from build123d import *

# Parameters (mm, degrees)
F0_R     = 5
F0_R_2   = 1.5
F0_R_3   = 2.5
F1_DEPTH = 5
F2_DEPTH = 45
F3_DEPTH = 4.7
F4_DEPTH = 20
F7_DEPTH = 15


with BuildPart() as f1:
    # F0 (on Front) → F1 (new body)
    with BuildSketch(Plane.XZ):
        with BuildLine():
            ThreePointArc((-17.146428, 3.5), (-16.612416, -5.502512), (-11.666667, -13.04373))
            ThreePointArc((-11.666667, -13.04373), (0, -17.5), (11.666667, -13.04373))
            ThreePointArc((11.666667, -13.04373), (16.612416, -5.502512), (17.146428, 3.5))
            ThreePointArc((17.146428, 3.5), (0, 17.5), (-17.146428, 3.5))
        make_face()
        Circle(F0_R, mode=Mode.SUBTRACT)
        with BuildLine():
            Line((-23.333333, -2.608746), (-11.666667, -13.04373))
            ThreePointArc((-11.666667, -13.04373), (-16.612416, -5.502512), (-17.146428, 3.5))
            Line((-17.146428, 3.5), (-21, 3.5))
            ThreePointArc((-21, 3.5), (-24.269603, 1.248877), (-23.333333, -2.608746))
        make_face()
        with Locations((-21, 0)):
            Circle(F0_R_2, mode=Mode.SUBTRACT)
        Circle(F0_R_3)
        with BuildLine():
            ThreePointArc((17.146428, 3.5), (16.612416, -5.502512), (11.666667, -13.04373))
            Line((11.666667, -13.04373), (23.333333, -2.608746))
            ThreePointArc((23.333333, -2.608746), (24.269603, 1.248877), (21, 3.5))
            Line((21, 3.5), (17.146428, 3.5))
        make_face()
        with Locations((21, 0)):
            Circle(F0_R_2, mode=Mode.SUBTRACT)
        Circle(F0_R)
        Circle(F0_R_3, mode=Mode.SUBTRACT)
    extrude(amount=-F1_DEPTH)

    # F0 (on Front) → F2 (join)
    with BuildSketch(Plane.XZ):
        with BuildLine():
            ThreePointArc((-17.146428, 3.5), (-16.612416, -5.502512), (-11.666667, -13.04373))
            ThreePointArc((-11.666667, -13.04373), (0, -17.5), (11.666667, -13.04373))
            ThreePointArc((11.666667, -13.04373), (16.612416, -5.502512), (17.146428, 3.5))
            ThreePointArc((17.146428, 3.5), (0, 17.5), (-17.146428, 3.5))
        make_face()
        Circle(F0_R, mode=Mode.SUBTRACT)
        Circle(F0_R)
        Circle(F0_R_3, mode=Mode.SUBTRACT)
        Circle(F0_R_3)
    extrude(amount=-F2_DEPTH)

    # F0 (on Front) → F3 (join)
    with BuildSketch(Plane.XZ):
        Circle(F0_R)
        Circle(F0_R_3, mode=Mode.SUBTRACT)
        Circle(F0_R_3)
    extrude(amount=F3_DEPTH)

    # F0 (on Front) → F4 (join)
    with BuildSketch(Plane.XZ):
        Circle(F0_R_3)
    extrude(amount=F4_DEPTH)


with BuildPart() as f1_1:
    # F5: moved
    add(f1.part.moved(Location((0, -43, 0))))

    # F6 (on Front) → F7 (join)
    with BuildSketch(Plane.XZ):
        Polygon((18.091601, 15.535572), (4.408399, 23.435572), (0.966088, 17.473313), (14.649289, 9.573313), align=None)
    extrude(amount=F7_DEPTH)


solid = f1_1.part
For this review, take the finished solid that the model builds, in its own axes (mm). A direction names the side the tool comes from. Give positions to 0.01 mm unless a question says otherwise; leave off trailing zeros. Loops run counter-clockwise (first coordinate to the right, second up) from the corner with the lowest first, then second, coordinate; pieces in that order, holes last. Notation, with made-up numbers: M 70.25,59.5 L 122.25,59.5 A21 ccw 122.25,68.5 Z; hole C 30.25,-22.75 d7. An arc over 180 degrees is marked long. Answer as a JSON object with one key per item and string values. Group by question number.
Q1. Mouldability with a two-part tool opening along X and no side actions: class faces 4 (the flat face through (9, -15, 17)), 5 (the flat face through (17.42, -40.53, -7.9)), 6 (the cylindrical face through (-22.5, -40.53, 0.07)) as +X half, -X half, draft (parallel to the pull), parting line (faces both ways), or undercut.
Q2. For probe 1 along Y at (x, z) = (6.5, -13); probe 2 along Y at (x, z) = (14, 11); probe 3 along Z at (x, y) = (21, -40), list the stretches that pass through material, from the lowest coordinate up. Write a range as [from, to].
Q3. Add section A-A on z = 0. Give the boundary of the cut face in (x, y).
Q4. Tool access review of faces 1 (the cylindrical face through (-1.08, -45.32, -4.88)), 2 (the flat face through (16.346, -7.395, 12.513)), 3 (the flat face through (19, -41, 3.5)): name each direction out of +Z, -Z, +X, -X, +Y, -Y from which nothing blocks a thin tool from reaching the whole face with its end or side.
Q5. Add section B-B on y = -14. Give the boundary of the cut face in (x, z).
Q6. Add section D-D on x = 16. Give the boundary of the cut face in (y, z), and give its area (3 significant figures).
Q7. Add section C-C on x = 0. Give the boundary of the cut face in (y, z).
Q8. Insertion check: P1, Ø1.9, axis at x = -18.5, y = -41.5, coming from the +Z side; P2, Ø4, axis at x = 21, z = 0, coming from the -Y side; P3, Ø12, axis at x = 7, y = -51.5, coming from the -Z side. Each pin has a flat end and moves straight along its axis. Give the tip position at first contact, or say it passes through.
Checked values:
{
 "1": {"face 4": "draft", "face 5": "+X half", "face 6": "undercut"},
 "2": {"probe 1": "[-43, 2]", "probe 2": "[-15, 0]", "probe 3": "[-4.7, -1.5], [1.5, 3.5]"},
 "3": {"outline": "M -24.5,-43 L -22.5,-43 L -22.5,-38 L -24.5,-38 Z; M -19.5,-43 L -5,-43 L -5,-47.7 L -2.5,-47.7 L -2.5,-63 L 2.5,-63 L 2.5,-47.7 L 5,-47.7 L 5,-43 L 19.5,-43 L 19.5,-38 L 17.5,-38 L 17.5,2 L -17.5,2 L -17.5,-38 L -19.5,-38 Z; M 22.5,-43 L 24.5,-43 L 24.5,-38 L 22.5,-38 Z"},
 "4": {"face 1": "-Y", "face 2": "+X, +Y, -Y", "face 3": "+Z, +X, +Y, -Y"},
 "5": {"outline": "M -11.67,-13.04 A17.5 ccw 11.67,-13.04 A17.5 ccw 14.65,9.57 L 18.09,15.54 L 4.41,23.44 L 0.97,17.47 A17.5 ccw Z"},
 "6": {"outline": "M -43,-9.17 L -38,-9.17 L -38,-7.09 L 2,-7.09 L 2,7.09 L -43,7.09 Z; M -15,11.91 L 0,11.91 L 0,16.74 L -15,16.74 Z", "area": "721 mm²"},
 "7": {"outline": "M -63,-2.5 L -47.7,-2.5 L -47.7,-5 L -43,-5 L -43,-17.5 L 2,-17.5 L 2,17.5 L -43,17.5 L -43,5 L -47.7,5 L -47.7,2.5 L -63,2.5 Z"},
 "8": {"P1": "z = 3.5", "P2": "y = -43", "P3": "z = -4.41"}
}
